Verification items for the finished model (mm, model axes). Face numbers are marked on the shaded views. A direction names the side the tool comes from. Round coordinates to 2 decimals unless told otherwise and drop trailing zeros. Write each loop counter-clockwise with the first axis right and the second up, starting at its lowest first coordinate (ties: lowest second). Pieces come first, ordered by that corner, then holes. Notation, with made-up numbers: (88, 80) - (116, 80) arc R25 ccw to (116, 104) - close; hole circle Ø5 at (32.25, -20.75). An arc over 180 degrees is marked (long way). Answer as a JSON object with one key per item and string values. Group by question number.
1) Section check A-A (z = 64). Enter the section's corners in (x, y).
2) Thickness scan on line 1 (Z direction, x = 35, y = 18); line 2 (Y direction, x = 12.5, z = 96); line 3 (X direction, y = 1.5, z = 40). Record the ranges inside material, lowest first.
3) Section check D-D (z = 50.5). Enter the section's corners in (x, y), then the cut area to 3 significant figures.
4) Go/stop test with flat-tipped pins: pin 1 Ø6 at (x, y) = (16.5, 10) entering from -Z; pin 2 Ø6 at (x, y) = (35, 2) entering from -Z. Record where each tip stops, or that it passes through.
5) Section check C-C (x = 33.5). Enter the section's corners in (y, z).
6) Set-up check for the marked faces 1 and 2: record each of +Z, -Z, +X, -X, +Y, -Y from which the full face is reachable in a straight line by a thin tool's end or side.
7) Section check B-B (y = 0). Enter the section's corners in (x, z).
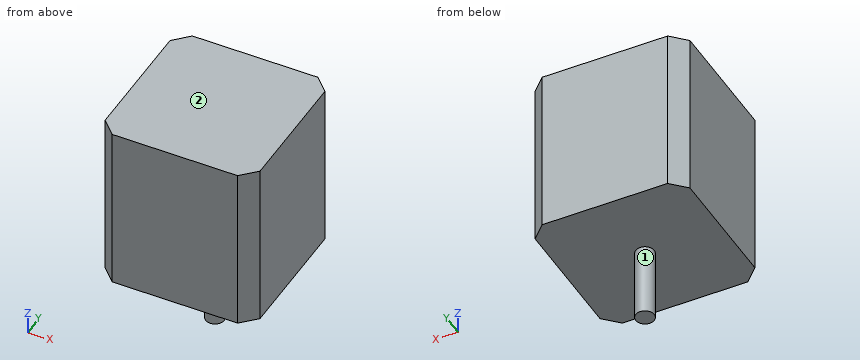
```python
from build123d import *

# Parameters (mm, degrees)
SKETCH_W     = 42
SKETCH_H     = 42
PAD_DEPTH    = 46
CHAMFER_SIZE = 4
SKETCH001_R  = 2.5
PAD001_DEPTH = 20


with BuildPart() as part:
    # Sketch → Pad (new body)
    with BuildSketch(Plane.XY):
        Rectangle(SKETCH_W, SKETCH_H)
    extrude(amount=PAD_DEPTH)

    # Chamfer
    chamfer_edges = [part.edges().sort_by_distance(p)[0] for p in [
        (-21, 21, 23),
        (-21, -21, 23),
        (21, -21, 23),
        (21, 21, 23),
    ]]
    chamfer(chamfer_edges, length=CHAMFER_SIZE)

    # Sketch001 → Pad001 (join)
    with BuildSketch(Plane.XY):
        Circle(SKETCH001_R)
    extrude(amount=-PAD001_DEPTH)


with BuildPart() as part_1:
    # Body placement: moved
    add(part.part.moved(Location((30, 0, 54))))


solid = part_1.part
```
Returned:
{
 "1": {"outline": "(9, -17) - (13, -21) - (47, -21) - (51, -17) - (51, 17) - (47, 21) - (13, 21) - (9, 17) - close"},
 "2": {"line 1": "54 to 100", "line 2": "-20.5 to 20.5", "line 3": "28 to 32"},
 "3": {"outline": "circle Ø5 at (30, 0)", "area": "19.6 mm2"},
 "4": {"pin 1": "z = 54", "pin 2": "z = 34"},
 "5": {"outline": "(-21, 54) - (21, 54) - (21, 100) - (-21, 100) - close"},
 "6": {"face 1": "-Z", "face 2": "+Z, +X, -X, +Y, -Y"},
 "7": {"outline": "(9, 54) - (27.5, 54) - (27.5, 34) - (32.5, 34) - (32.5, 54) - (51, 54) - (51, 100) - (9, 100) - close"}
}
